Input: part model. Units: mm. Frame: model coordinates. A direction names the side the tool comes from. Coordinates: 2 decimals unless noted, no trailing zeros. Order: outer loops, then holes, each group sorted by start corner. A loop starts at its lowest first (then second) coordinate and runs counter-clockwise, first axis right, second up. Notation, with made-up numbers: (3, 40.25) -> (16, 40.25) arc R29 cw to (16, 69.25) -> close; hole circle Ø3 at (75.25, 3.25). An arc over 180 degrees is marked (long way). Use one line per item in the form item = value. Start each with the question number.
1) Section query D-D on x = -33. Output: boundary loops of the cut face in (y, z).
2) Ray query, line 1 along Y through (x, z) = (-2, -15); line 2 along Z through (x, y) = (-14, 10); line 3 along Y through (x, z) = (-21.75, -15). Return the intervals inside material, ascending.
3) Section query C-C on y = 30. Count the separate pieces of the cut face and the enclosed holes in it, then the cut area to 3 significant figures.
4) Section query B-B on z = -28. Output: boundary loops of the cut face in (x, y), then the cut area to 3 significant figures.
5) Access query for faces 1 (the cylindrical face through (-23.79, 27.95, -14.54)), 2 (the conical face through (-18.14, 30.1, -19.64)), 3 (the flat face through (-29.5, 40, -5)). Directions: +Z, -Z, +X, -X, +Y, -Y. A direction counts if a zero-diameter tool reaches every point of the face in a straight line with its end or side. Return the directions, or none.
6) Draft query along Z for faces 4 (the conical face through (-18.14, 29.9, 19.64)), 5 (the flat face through (0, 15.4, -11.3)), 6 (the cylindrical face through (-17.26, -18.81, -10.84)). Return one class per face: pulls with the +Z half, pulls with the -Z half, needs draft (parallel to the pull), parting line crosses it, or undercut.
7) Pin query (flat end, axial travel): pin 1 (1.5 mm diameter, centred on y = 18.5, z = -1.5, fed in from +X); pin 2 (4 mm diameter, centred on y = 42, z = 32.5, fed in from -X); pin 3 (8 mm diameter, centred on x = -30.5, y = 53.5, fed in from +Z). Return the tip coordinate at first contact, or that it passes through.
from build123d import *

# Parameters (mm, degrees)
CUT_EXTRUDE_START        = -11
CUT_EXTRUDE_1_DEPTH      = 11
CUT_EXTRUDE_2_DEPTH      = 27
EXTRUDE_START            = -1
SKETCH_4_R               = 50
SKETCH_4_R_2             = 6.5
EXTRUDE_1_DEPTH          = 1
EXTRUDE_2_DEPTH          = 6
EXTRUDE_2_DEPTH_BACK     = 29
SKETCH_5_R               = 50
SKETCH_5_R_2             = 49
EXTRUDE_3_DEPTH          = 1.5
EXTRUDE_3_DEPTH_BACK     = 10
SKETCH_15_R              = 12
SKETCH_15_R_2            = 11
EXTRUDE_4_DEPTH          = 10
M5X0_81_D                = 4.2
M5X0_81_CSINK_D          = 5.05
M5X0_81_CSINK_ANGLE      = 90
FILLET_1_R               = 2
FILLET_1_OF_MIRROR_1_R   = 2
FILLET_2_R               = 1
CHAMFER_1_SIZE           = 0.5
CUT_EXTRUDE_4_DEPTH      = 99.40731683
CUT_EXTRUDE_4_DEPTH_BACK = 99.40731683
SKETCH_16_R              = 11
CUT_EXTRUDE_3_REACH      = 100.697
SKETCH_12_R              = 5
M2X0_41_D                = 1.6
PATTERN_CIRCULAR_1_COUNT = 3


with BuildPart() as part:
    # Эскиз1 → Повернуть1 (revolve)
    with BuildSketch(Plane.XY, mode=Mode.PRIVATE) as revolve_1_sk:
        Polygon((-27, 7.5), (-27, 8.5), (-28, 8.5), (-28, 18), (-7, 18), (-7, 18.5), (0, 18.5), (0, 19.5), (-29, 19.5), (-29, 6.5), (-22, 6.5), (-22, 7.5), align=None)
    revolve(revolve_1_sk.sketch.rotate(Axis((0, 0, 0), (1, 0, 0)), 90), axis=Axis((0, 0, 0), (1, 0, 0)))

    # Эскиз2 → Вырез-Вытянуть1 (cut)
    with BuildSketch(Plane(origin=(0, 0, 0), x_dir=(0, 0, -1), z_dir=(1, 0, 0)).offset(CUT_EXTRUDE_START)):
        with BuildLine():
            Line((5.156251293, 18.805931846), (5, 16.248076809))
            ThreePointArc((5, 16.248076809), (-12.02081528, 12.02081528), (-16.248076809, -5))
            Line((-16.248076809, -5), (-18.848076825, -5))
            ThreePointArc((-18.848076825, -5), (-13.731246096, 13.845680938), (5.156251293, 18.805931846))
        make_face()
    extrude(amount=CUT_EXTRUDE_1_DEPTH, mode=Mode.SUBTRACT)

    # Эскиз3 → Вырез-Вытянуть2 (cut)
    with BuildSketch(Plane(origin=(0, 0, 0), x_dir=(0, 0, -1), z_dir=(1, 0, 0))):
        with BuildLine():
            Line((-40, 11.5), (-12.519984026, 11.5))
            ThreePointArc((-12.519984026, 11.5), (-9.954045186, 13.781037132), (-6.982120022, 15.5))
            Line((-6.982120022, 15.5), (-13.240816858, 29.394032278))
            Line((-13.240816858, 29.394032278), (-40, 11.5))
        make_face()
    extrude(amount=-CUT_EXTRUDE_2_DEPTH, mode=Mode.SUBTRACT)

    # Эскиз4 → Бобышка-Вытянуть1 (add)
    with BuildSketch(Plane.ZY.offset(29).offset(EXTRUDE_START)):
        with Locations((0, 30)):
            Circle(SKETCH_4_R)
        Circle(SKETCH_4_R_2, mode=Mode.SUBTRACT)
    extrude(amount=EXTRUDE_1_DEPTH)

    # Эскиз5 → Бобышка-Вытянуть2 (add, two sides: drawn at the far end of the back side and taken through both)
    with BuildSketch(Plane.ZY.offset(29).offset(-EXTRUDE_2_DEPTH_BACK)):
        with Locations((0, 30)):
            Circle(SKETCH_5_R)
        with Locations(Location((0, 30, 0), (0, 0, 180))):
            Circle(SKETCH_5_R_2, mode=Mode.SUBTRACT)
    extrude(amount=EXTRUDE_2_DEPTH + EXTRUDE_2_DEPTH_BACK)

    # Эскиз15 → Бобышка-Вытянуть3 (add, two sides: drawn at the far end of the back side and taken through both)
    with BuildSketch(Plane.ZY.offset(28).offset(-EXTRUDE_3_DEPTH_BACK)):
        with Locations(Location((0, 30, 0), (0, 0, 180))):
            Circle(SKETCH_15_R)
        with Locations(Location((0, 30, 0), (0, 0, 180))):
            Circle(SKETCH_15_R_2, mode=Mode.SUBTRACT)
    extrude(amount=EXTRUDE_3_DEPTH + EXTRUDE_3_DEPTH_BACK)

    # Эскиз17 → Бобышка-Вытянуть4 (add)
    with BuildSketch(Plane(origin=(-28, 0, 0), x_dir=(0, 0, -1), z_dir=(1, 0, 0))):
        with BuildLine():
            Line((-15, 35), (-10.908712115, 35))
            ThreePointArc((-10.908712115, 35), (-12, 30), (-10.908712115, 25))
            Line((-10.908712115, 25), (-15, 25))
            ThreePointArc((-15, 25), (-20, 30), (-15, 35))
        make_face()
    extrude_4 = extrude(amount=EXTRUDE_4_DEPTH)

    # Отверстие обработанное метчиком M5x0.81 (through all)
    with Locations(Plane(origin=(-18, 0, 0), x_dir=(0, 0, -1), z_dir=(1, 0, 0))):
        with Locations((-15, 30)):
            m5x0_81 = CounterSinkHole(M5X0_81_D / 2, M5X0_81_CSINK_D / 2, counter_sink_angle=M5X0_81_CSINK_ANGLE)

    # Скругление1
    fillet_1_edges = [part.edges().sort_by_distance(p)[0] for p in [
        (-23, 25, 10.908712115),
        (-23, 35, 10.908712115),
    ]]
    fillet(fillet_1_edges, radius=FILLET_1_R)

    # Зеркальное отражение1: Бобышка-Вытянуть4, Отверстие обработанное метчиком M5x0.81 across plane
    add(extrude_4.mirror(Plane.XY))
    add(m5x0_81.mirror(Plane.XY), mode=Mode.SUBTRACT)

    # Скругление1 of Зеркальное отражение1
    fillet_1_of_mirror_1_edges = [part.edges().sort_by_distance(p)[0] for p in [
        (-23, 25, -10.908712115),
        (-23, 35, -10.908712115),
    ]]
    fillet(fillet_1_of_mirror_1_edges, radius=FILLET_1_OF_MIRROR_1_R)

    # Скругление2
    fillet_2_edges = [part.edges().sort_by_distance(p)[0] for p in [
        (-28, 20.998545842, -7.935604769),
        (-28, 30, 20),
        (-28, 25, 13.562177826),
        (-28, 20.998545842, 7.935604769),
        (-28, 35, 13.562177826),
        (-28, 35.267949192, 11.124355653),
        (-28, 24.732050808, 11.124355653),
        (-28, 30, -20),
        (-28, 25, -13.562177826),
        (-28, 42, 0),
        (-28, 35, -13.562177826),
        (-28, 35.267949192, -11.124355653),
        (-28, 24.732050808, -11.124355653),
    ]]
    fillet(fillet_2_edges, radius=FILLET_2_R)

    # Фаска1
    chamfer_1_edges = [part.edges().sort_by_distance(p)[0] for p in [
        (-18, 20.998545842, 7.935604769),
        (-18, 30, 20),
        (-18, 25, 13.562177826),
        (-18, 35, 13.562177826),
        (-18, 42, 0),
        (-18, 24.732050808, 11.124355653),
        (-18, 35.267949192, 11.124355653),
        (-18, 30, -20),
        (-18, 25, -13.562177826),
        (-18, 20.998545842, -7.935604769),
        (-18, 35, -13.562177826),
        (-18, 24.732050808, -11.124355653),
        (-18, 35.267949192, -11.124355653),
    ]]
    chamfer(chamfer_1_edges, length=CHAMFER_1_SIZE)

    # Эскиз16 → Вырез-Вытянуть4 (cut, two sides: drawn at the far end of the back side and taken through both)
    with BuildSketch(Plane(origin=(-28, 0, 0), x_dir=(0, 0, -1), z_dir=(1, 0, 0)).offset(-CUT_EXTRUDE_4_DEPTH_BACK)):
        with Locations(Location((0, 30, 0), (0, 0, 283.872102735))):
            Circle(SKETCH_16_R)
    extrude(amount=CUT_EXTRUDE_4_DEPTH + CUT_EXTRUDE_4_DEPTH_BACK, mode=Mode.SUBTRACT)

    # Эскиз12 → Вырез-Вытянуть3 (cut, up to next)
    with BuildSketch(Plane.ZY.offset(29), mode=Mode.PRIVATE) as cut_extrude_3_sk1:
        with Locations((0, 56.4)):
            Circle(SKETCH_12_R)
    cut_extrude_3_tool1 = extrude(cut_extrude_3_sk1.sketch, amount=-CUT_EXTRUDE_3_REACH, mode=Mode.PRIVATE) & part.part
    add(cut_extrude_3_tool1.solids().sort_by_distance((-29, 56.4, 0))[0], mode=Mode.SUBTRACT)

    # Сверление под метчик M2x0.41 (through all)
    with Locations(Plane.ZY.offset(29)):
        with Locations((0, 62.9)):
            m2x0_41 = Hole(M2X0_41_D / 2)

    # Круговой массив1: Сверление под метчик M2x0.41 ×3 about axis
    pattern_circular_1_axis = Axis((0, 56.4, 0), (1, 0, 0))
    for i in range(1, PATTERN_CIRCULAR_1_COUNT):
        add(m2x0_41.rotate(pattern_circular_1_axis, i * 360 / PATTERN_CIRCULAR_1_COUNT), mode=Mode.SUBTRACT)


solid = part.part
Answers below:
q1.outline = circle Ø100 at (30, 0); hole circle Ø98 at (30, 0)
q2.line_1 = -17.7 to -16.65, -12.46 to -10.83, 10.83 to 12.46, 76.65 to 77.7
q2.line_2 = -45.83 to -44.73, -16.74 to -14.97, 14.97 to 16.74, 44.73 to 45.83
q2.line_3 = -17.7 to -16.65, -12.46 to -9.95, 9.95 to 12.46, 25 to 27.9, 32.1 to 35, 76.65 to 77.7
q3.separate_pieces = 4
q3.enclosed_holes = 0
q3.area = 234 mm^2
q4.outline = (-35, -11.42) -> (0, -11.42) -> (0, -10.21) -> (-28, -10.21) -> (-28, 70.21) -> (0, 70.21) -> (0, 71.42) -> (-35, 71.42) -> (-35, 70.21) -> (-29, 70.21) -> (-29, -10.21) -> (-35, -10.21) -> close
q4.area = 165 mm^2
q5.face_1 = +X, -X
q5.face_2 = +X
q5.face_3 = -X
q6.face_4 = undercut
q6.face_5 = needs draft
q6.face_6 = parting line crosses it
q7.pin_1 = -11
q7.pin_2 = -29
q7.pin_3 = 46.04
